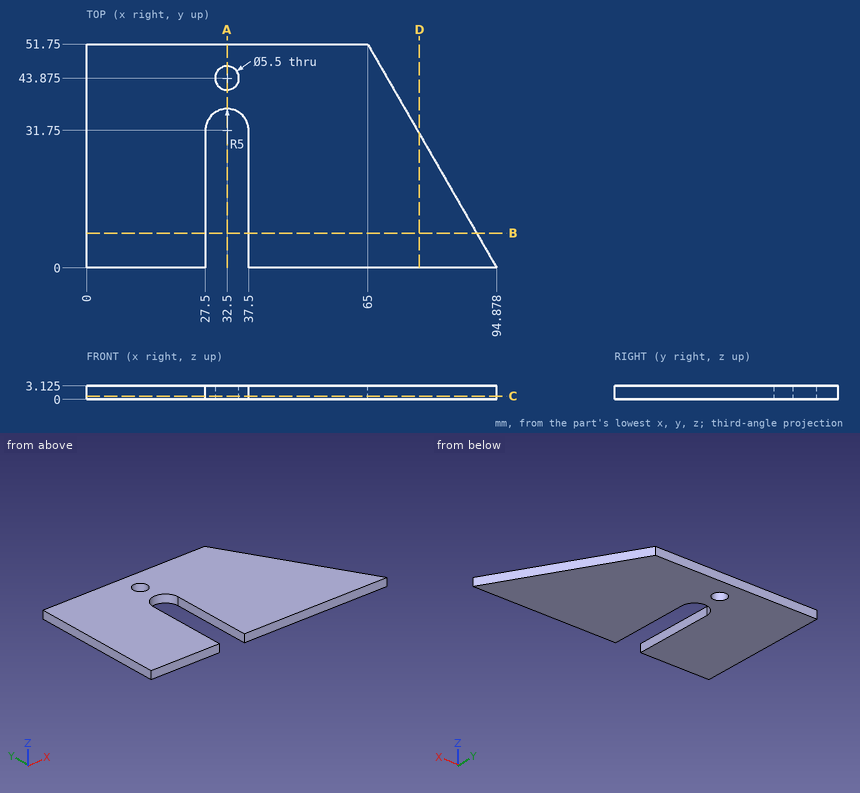
Design review of the part shown in the three views and the two pictorial views. Dimensions are in mm from the part's minimum x, y and z. Round coordinates to 2 decimals unless told otherwise and drop trailing zeros. Write each loop counter-clockwise with the first axis right and the second up, starting at its lowest first coordinate (ties: lowest second). Pieces come first, ordered by that corner, then holes.
Item 1: We need section C-C on z = 0.75. Write out the cut boundary in (x, y) (3 decimals), and give its area (3 significant figures).
Item 2: We need section B-B on y = 8. Write out the cut boundary in (x, z) (3 decimals).
Item 3: For probe 1 along Y at (x, z) = (32.5, 1.45) (3 decimals); probe 2 along X at (y, z) = (6, 0.4); probe 3 along X at (y, z) = (13, 2.05), list the stretches that pass through material, from the lowest coordinate up.
Item 4: We need section A-A on x = 32.5. Write out the cut boundary in (y, z) (3 decimals).
Item 5: We need section D-D on x = 77. Write out the cut boundary in (y, z) (1 decimal).
Item 6: Clearance check with flat-ended pins moving along their axes: pin 1 Ø3.5 at (x, y) = (32.5, 43.875) entering from +Z; pin 2 Ø1.6 at (y, z) = (15.5, 1) entering from +X. State where each tip first meets the part, or that it passes through.
Returned:
1. outline: (0, 0) - (27.5, 0) - (27.5, 31.75) arc R5 cw to (37.5, 31.75) - (37.5, 0) - (94.878, 0) - (65, 51.75) - (0, 51.75) - close; hole circle Ø5.5 at (32.5, 43.875)
1. area: 3,760 mm2
2. outline: (0, 0) - (27.5, 0) - (27.5, 3.125) - (0, 3.125) - close; (37.5, 0) - (90.259, 0) - (90.259, 3.125) - (37.5, 3.125) - close
3. probe 1: y = 36.75 to 41.125, 46.625 to 51.75
3. probe 2: x = 0 to 27.5, 37.5 to 91.41
3. probe 3: x = 0 to 27.5, 37.5 to 87.37
4. outline: (36.75, 0) - (41.125, 0) - (41.125, 3.125) - (36.75, 3.125) - close; (46.625, 0) - (51.75, 0) - (51.75, 3.125) - (46.625, 3.125) - close
5. outline: (0, 0) - (31, 0) - (31, 3.1) - (0, 3.1) - close
6. pin 1: passes through
6. pin 2: stops at x = 86.39
